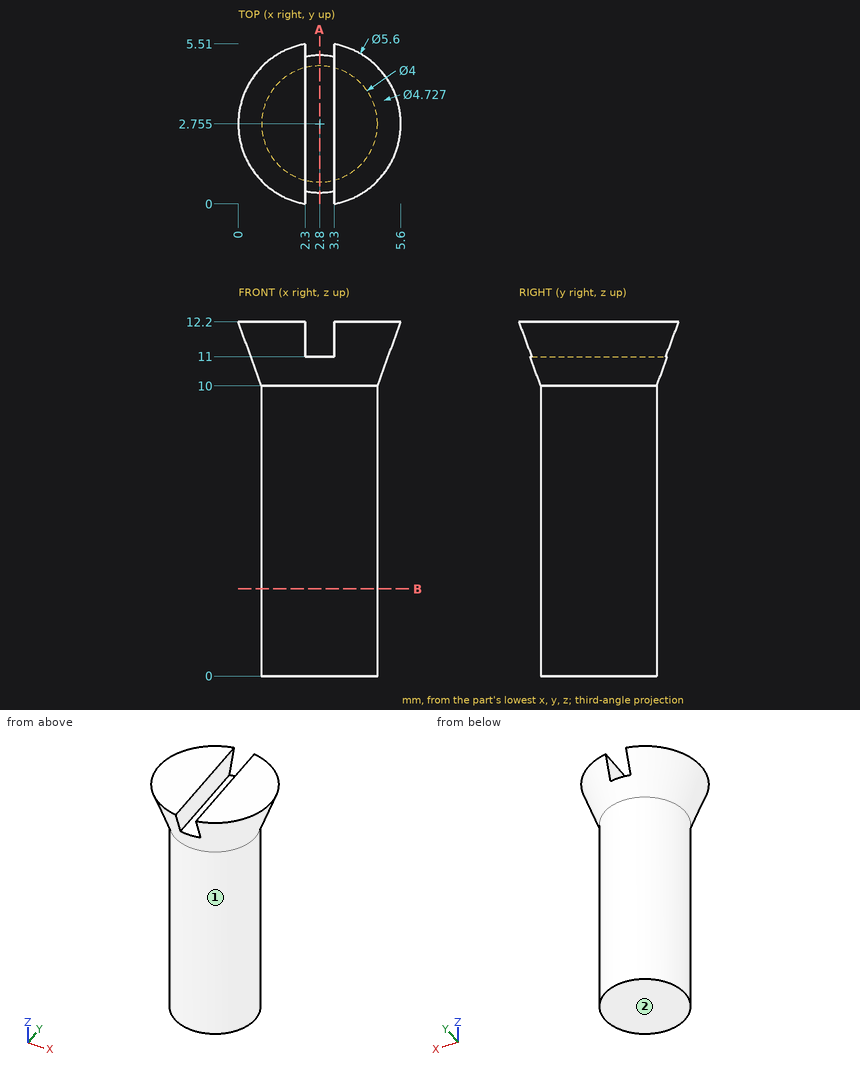
Here's the drawing with two shaded views (mm, measured from the low corner). I have some questions. A direction names the side the tool comes from. Give positions to 0.01 mm unless a question says otherwise; leave off trailing zeros. Write each loop counter-clockwise with the first axis right and the second up, starting at its lowest first coordinate (ties: lowest second). Pieces come first, ordered by that corner, then holes. Notation, with made-up numbers: (-33, -40) - (-11, -40) arc R20 ccw to (-11, -9) - close; hole circle Ø1 at (54.5, 84.5). An arc over 180 degrees is marked (long way). Write item = value, one per line. Start each with the question number.
1. For pin 1 (1.5 mm diameter, centred on y = 4, z = 1.5, fed in from -X); pin 2 (1 mm diameter, centred on x = 3.5, z = 2.5, fed in from -Y) (3 decimals); pin 3 (0.6 mm diameter, centred on y = 2.5, z = 11.5, fed in from +X) (1 decimal), each with a flat end and sliding along its axis, tell me the tip position at first contact or that it passes through.
2. Please list where these lines run through material, in increasing order: line 1 (X direction, y = 2.65, z = 2); line 2 (Y direction, x = 2.75, z = 8); line 3 (Z direction, x = 2.75, y = 2.2).
3. Imagine slicing it at A-A (x = 2.8). Please give me the cut outline in (y, z) (1 decimal).
4. On a 3-axis mill with a long thin cutter (end or side, diameter ignored), from which of +Z, -Z, +X, -X, +Y, -Y can I reach the whole of each face in a straight line? I mean the marked faces 1 and 2. Say none if no direction works.
5. Imagine slicing it at B-B (z = 3). Please give me the cut outline in (x, y) (1 decimal).
Worked answers:
q1.pin_1 = 0.86
q1.pin_2 = 0.765
q1.pin_3 = 5.4
q2.line_1 = 0.8 to 4.8
q2.line_2 = 0.76 to 4.75
q2.line_3 = 0 to 11
q3.outline = (0.4, 11) - (0.8, 10) - (0.8, 0) - (4.8, 0) - (4.8, 10) - (5.1, 11) - close
q4.face_1 = -Z
q4.face_2 = -Z, +X, -X, +Y, -Y
q5.outline = circle Ø4 at (2.8, 2.8)
